from build123d import *

# Parameters (mm, degrees)
F1_DEPTH  = 9.525
F3_DEPTH  = 30.48
F4_R      = 3.556
F5_DEPTH  = 36.195
F7_DEPTH  = 12.7
F8_R      = 1.5875
F9_R      = 1.905
F10_DEPTH = 19.05


# Not quite as in the source:
# - a feature names something its author has since deleted; it is built from what else it names


with BuildPart() as f1:
    # F0 (on Front) → F1 (new body, symmetric)
    with BuildSketch(Plane.XZ):
        Polygon((-31.75, 50.8), (-31.75, 0), (-6.35, 0), (-5.08, 15.875), (0, 15.875), (0, 66.675), (-19.05, 66.675), align=None)
        Polygon((19.05, 66.675), (0, 66.675), (0, 15.875), (5.08, 15.875), (6.35, 0), (31.75, 0), (31.75, 50.8), align=None)
    extrude(amount=F1_DEPTH, both=True)

    # F2 (on face) → F3 (cut)
    with BuildSketch(Plane.XY.offset(66.675)):
        with BuildLine():
            Line((26.67, -4.0005), (26.67, 4.0005))
            Line((26.67, 4.0005), (3.7759814618, 4.0005))
            ThreePointArc((3.7759814618, 4.0005), (0, 6.1595), (-3.7759814618, 4.0005))
            Line((-3.7759814618, 4.0005), (-26.67, 4.0005))
            Line((-26.67, 4.0005), (-26.67, -4.0005))
            Line((-26.67, -4.0005), (26.67, -4.0005))
        make_face()
        with BuildLine():
            ThreePointArc((26.67, -4.0005), (29.2644515955, 0), (26.67, 4.0005))
            Line((26.67, 4.0005), (26.67, -4.0005))
        make_face()
        with BuildLine():
            ThreePointArc((-26.67, 4.0005), (-29.2644515955, 0), (-26.67, -4.0005))
            Line((-26.67, -4.0005), (-26.67, 4.0005))
        make_face()
    extrude(amount=-F3_DEPTH, mode=Mode.SUBTRACT)

    # F4 (on Top) → F5 (cut, through all)
    with BuildSketch(Plane.XY):
        Circle(F4_R)
    extrude(amount=F5_DEPTH, mode=Mode.SUBTRACT)

    # F6 (on Front) → F7 (cut, symmetric)
    with BuildSketch(Plane.XZ):
        Polygon((-8.89, 33.5468458159), (-26.9126990667, 33.5468458159), (-26.9126990667, 6.7006074823), (-11.0376990667, 6.7006074823), align=None)
        Polygon((8.89, 33.5468458159), (11.0376990667, 6.7006074823), (26.9126990667, 6.7006074823), (26.9126990667, 33.5468458159), align=None)
    extrude(amount=F7_DEPTH, both=True, mode=Mode.SUBTRACT)

    # F8
    f8_edges = [f1.edges().sort_by_distance(p)[0] for p in [
        (31.75, 9.525, 25.4),
        (25.4, 9.525, 58.7375),
        (31.75, -9.525, 25.4),
        (25.4, -9.525, 58.7375),
        (5.715, 9.525, 7.9375),
        (5.715, -9.525, 7.9375),
        (-5.715, -9.525, 7.9375),
        (-5.715, 9.525, 7.9375),
        (-31.75, 9.525, 25.4),
        (-31.75, -9.525, 25.4),
        (-25.4, 9.525, 58.7375),
        (-25.4, -9.525, 58.7375),
        (-17.90135, 9.525, 33.546846),
        (-26.912699, 9.525, 20.123727),
        (-18.975199, 9.525, 6.700607),
        (-9.96385, 9.525, 20.123727),
        (9.96385, 9.525, 20.123727),
        (18.975199, 9.525, 6.700607),
        (26.912699, 9.525, 20.123727),
        (17.90135, 9.525, 33.546846),
        (-17.90135, -9.525, 33.546846),
        (-26.912699, -9.525, 20.123727),
        (-18.975199, -9.525, 6.700607),
        (-9.96385, -9.525, 20.123727),
        (9.96385, -9.525, 20.123727),
        (18.975199, -9.525, 6.700607),
        (26.912699, -9.525, 20.123727),
        (17.90135, -9.525, 33.546846),
    ]]
    fillet(f8_edges, radius=F8_R)

    # F9 (on face) → F10 (cut, through all)
    with BuildSketch(Plane(origin=(0, 9.525, 0), x_dir=(-1, 0, 0), z_dir=(0, 1, 0))):
        with Locations((-12.7, 47.625)):
            Circle(F9_R)
        with Locations((12.7, 47.625)):
            Circle(F9_R)
    extrude(amount=-F10_DEPTH, mode=Mode.SUBTRACT)


solid = f1.part
The listing builds one solid part. Answer for the finished solid, in the listing's coordinates (mm). A direction names the side the tool comes from. Coordinates: 2 decimals unless noted, no trailing zeros. Order: outer loops, then holes, each group sorted by start corner. A loop starts at its lowest first (then second) coordinate and runs counter-clockwise, first axis right, second up. Notation, with made-up numbers: M -12,-14 L 20,-14 A30 cw 20,12 Z; hole C 18.25,64 d1. An arc over 180 degrees is marked long. Use CSV: the item, a comma, the result in double quotes.
Q1. A tool of negligible diameter and unlimited length cuts with its end or side. For faces 1 (the cylindrical face through (-27.39, -9.07, 20.33)), 2 (the cylindrical face through (19.169, 9.072, 6.223)), 3 (the flat face through (-9.98, 0.11, 19.94)), 4 (the cylindrical face through (6.2, 9.07, 7.8)), 5 (the cylindrical face through (29.264, -0.071, 46.819)), from which of +Z, -Z, +X, -X, +Y, -Y can it reach the whole face along a straight path? Write none if from no direction.
Here are the results:
face 1,"-Y"
face 2,"+Y"
face 3,"+Y, -Y"
face 4,"-Z, +Y"
face 5,"+Z"
Q2. Section B-B (y = 0) is taken. Determine the outline of the cut face in (x, z) (3 decimals).
Here are the results:
outline,"M -31.75,0 L -6.35,0 L -5.08,15.875 L -3.556,15.875 L -3.556,36.195 L -29.264,36.195 L -29.264,53.907 L -31.75,50.8 Z; M 3.556,15.875 L 5.08,15.875 L 6.35,0 L 31.75,0 L 31.75,50.8 L 29.264,53.907 L 29.264,36.195 L 3.556,36.195 Z; hole M -26.913,6.701 L -11.038,6.701 L -8.89,33.547 L -26.913,33.547 Z; hole M 8.89,33.547 L 11.038,6.701 L 26.913,6.701 L 26.913,33.547 Z"
Q3. Given pin 1 Ø3 at (x, y) = (-10, 0) entering from +Z (3 decimals), flat-ended and moving along its own axis, determine where the tip first touches the part or whether it passes through.
Here are the results:
pin 1,"z = 36.195"
Q4. Determine the mould class of faces 6 (the cylindrical face through (-6.187, 9.072, 8.024)), 7 (the flat face through (0, -9.525, 41)), 8 (the cylindrical face through (9.495, 9.072, 20.002)) for opening direction Z: pulls with the +Z half, pulls with the -Z half, needs draft (parallel to the pull), parting line crosses it, or undercut.
Here are the results:
face 6,"pulls with the -Z half"
face 7,"needs draft"
face 8,"undercut"
Q5. Straight lines are drawn through the part: L1, parallel to Y at x = -12, z = 53 (1 decimal); L2, parallel to X at y = -5, z = 13; L3, parallel to Z at x = 18, y = -3.5 (3 decimals). For each, find the intervals that lie inside material, in ascending order.
Here are the results:
L1,"-9.5 to -4, 4 to 9.5"
L2,"-31.75 to -26.91, -10.53 to -5.31, 5.31 to 10.53, 26.91 to 31.75"
L3,"0 to 6.701, 33.547 to 36.195"
Q6. Section A-A (x = 12.7) is taken. Determine the outline of the cut face in (y, z) (1 decimal), then the cut area to 3 significant figures.
Here are the results:
outline,"M -9.5,0 L 9.5,0 L 9.5,5.1 A1.6 ccw 7.9,6.7 L -7.9,6.7 A1.6 ccw -9.5,5.1 Z; M -9.5,35.1 A1.6 ccw -7.9,33.5 L 7.9,33.5 A1.6 ccw 9.5,35.1 L 9.5,45.7 L 4,45.7 L 4,36.2 L -4,36.2 L -4,45.7 L -9.5,45.7 Z; M -9.5,49.5 L -4,49.5 L -4,66.7 L -9.5,66.7 Z; M 4,49.5 L 9.5,49.5 L 9.5,66.7 L 4,66.7 Z"
area,"471 mm2"
Q7. Section D-D (y = -7) is taken. Determine the outline of the cut face in (x, z) (3 decimals).
Here are the results:
outline,"M -31.75,0 L -6.35,0 L -5.08,15.875 L 5.08,15.875 L 6.35,0 L 31.75,0 L 31.75,50.8 L 19.05,66.675 L -19.05,66.675 L -31.75,50.8 Z; hole M -26.913,6.701 L -11.038,6.701 L -8.89,33.547 L -26.913,33.547 Z; hole C -12.7,47.625 d3.81; hole M 8.89,33.547 L 11.038,6.701 L 26.913,6.701 L 26.913,33.547 Z; hole C 12.7,47.625 d3.81"
